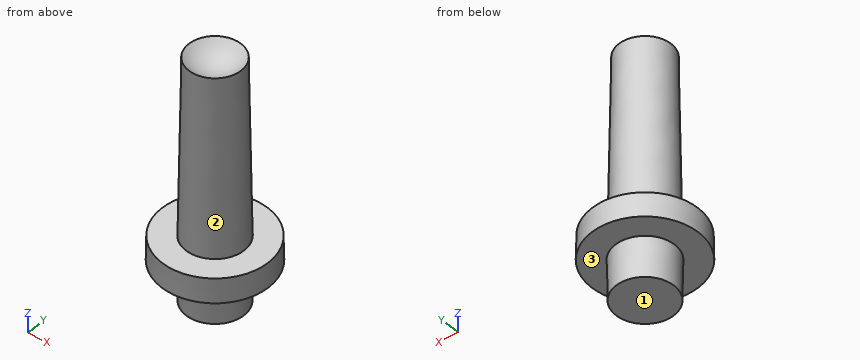
from build123d import *

# Parameters (mm, degrees)
SKETCH1_R           = 2.794
BOSS_EXTRUDE1_DEPTH = 1.27
BOSS_EXTRUDE1_TAPER = 1
SKETCH2_R           = 1.524
BOSS_EXTRUDE2_DEPTH = 9.23000005
BOSS_EXTRUDE2_TAPER = 1
SKETCH3_R           = 1.549999948
BOSS_EXTRUDE3_DEPTH = 2.1
BOSS_EXTRUDE3_TAPER = 1


with BuildPart() as part:
    # Sketch1 → Boss-Extrude1 (new body)
    with BuildSketch(Plane.XY):
        Circle(SKETCH1_R)
    extrude(amount=BOSS_EXTRUDE1_DEPTH, taper=BOSS_EXTRUDE1_TAPER)

    # Sketch2 → Boss-Extrude2 (add)
    with BuildSketch(Plane.XY.offset(1.27)):
        Circle(SKETCH2_R)
    extrude(amount=BOSS_EXTRUDE2_DEPTH, taper=BOSS_EXTRUDE2_TAPER)

    # Sketch3 → Boss-Extrude3 (add)
    with BuildSketch(Plane(origin=(0, 0, 0), x_dir=(-1, 0, 0), z_dir=(0, 0, -1))):
        Circle(SKETCH3_R)
    extrude(amount=BOSS_EXTRUDE3_DEPTH, taper=BOSS_EXTRUDE3_TAPER)

    # Sketch5 → Cut-Revolve4 (revolve, cut)
    with BuildSketch(Plane(origin=(0, 0, 0), x_dir=(1, 0, 0), z_dir=(0, 1, 0))):
        with BuildLine():
            Line((0, -10.50000005), (0, -9.94120005))
            ThreePointArc((0, -9.94120005), (0.736499476, -10.086324189), (1.36288975, -10.50000005))
            Line((1.36288975, -10.50000005), (1.36288975, -10.823922581))
            Line((1.36288975, -10.823922581), (0, -10.823922581))
            Line((0, -10.823922581), (0, -10.50000005))
        make_face()
    revolve(axis=Axis((0, 0, 1.27), (0, 0, 1)), mode=Mode.SUBTRACT)


solid = part.part
For this review, take the finished solid that the model builds, in its own axes (mm). Face numbers are marked on the shaded views. A direction names the side the tool comes from. Coordinates: 2 decimals unless noted, no trailing zeros. Order: outer loops, then holes, each group sorted by start corner. A loop starts at its lowest first (then second) coordinate and runs counter-clockwise, first axis right, second up. Notation, with made-up numbers: (-19.5, -7.5) - (8.5, -7.5) arc R22 ccw to (8.5, 21.5) - close; hole circle Ø11 at (-18, 28.5). An arc over 180 degrees is marked (long way). Answer as CSV lines item,"result". Start each with the question number.
1) Machinability: for the marked faces 1, 2 and 3, which of the approach directions +Z, -Z, +X, -X, +Y, -Y give a long, thin tool a straight path to every point of the face, cutting with its end or side? Answer none if there is none.
2) Add section A-A (z = -1). State the section outline as (x, y) points, then the cut area to 3 significant figures.
3) Add section B-B (z = 6.75). State the section outline as (x, y) points, then the cut area to 3 significant figures.
4) To check wall thickness, follow line 1 along Z through (x, y) = (-1.5, -2.1); line 2 along Z through (x, y) = (0.15, 0.7); line 3 along Y through (x, z) = (0.8, -0.5). State the ranges of each line that lie inside material, in increasing order. Write a range as [from, to].
Result:
1,face 1,"-Z, +X, -X, +Y, -Y"
1,face 2,"+Z"
1,face 3,"-Z"
2,outline,"circle Ø3.07 at (0, 0)"
2,area,"7.38 mm^2"
3,outline,"circle Ø2.86 at (0, 0)"
3,area,"6.41 mm^2"
4,line 1,"[0, 1.27]"
4,line 2,"[-2.1, 10.08]"
4,line 3,"[-1.32, 1.32]"
